from build123d import *

# Parameters (mm, degrees)
F2_R     = 2.54
F4_DEPTH = 3.81
F5_DEPTH = 5.08


with BuildPart() as f1:
    # F0 (on Front) → F1 (revolve)
    with BuildSketch(Plane.XZ):
        Polygon((0, 0), (0, 45.974), (-9.660285, 45.974), (-9.660285, 39.017074), (-6.224093, 36.049455), (-6.224093, 9.1948), (-8.699501, 9.1948), (-10.9982, 0), align=None)
    revolve(axis=Axis((0, 0, 22.987), (0, 0, 1)))

    # F2
    f2_edges = [f1.edges().sort_by_distance(p)[0] for p in [
        (8.699501, 0, 9.1948),
    ]]
    fillet(f2_edges, radius=F2_R)

    # F3 (on face) → F4 (cut)
    with BuildSketch(Plane.XY.offset(45.974)):
        with BuildLine():
            ThreePointArc((-5.499261, 3.175), (-4.490128, 4.490128), (-3.175, 5.499261))
            Line((-3.175, 5.499261), (-4.830143, 8.366052))
            ThreePointArc((-4.830143, 8.366052), (-6.830853, 6.830853), (-8.366052, 4.830143))
            Line((-8.366052, 4.830143), (-5.499261, 3.175))
        make_face()
        with BuildLine():
            ThreePointArc((0, 6.35), (1.643501, 6.133629), (3.175, 5.499261))
            Line((3.175, 5.499261), (4.830143, 8.366052))
            ThreePointArc((4.830143, 8.366052), (2.500266, 9.331119), (0, 9.660285))
            Line((0, 9.660285), (0, 6.35))
        make_face()
        with BuildLine():
            ThreePointArc((5.499261, 3.175), (6.133629, 1.643501), (6.35, 0))
            Line((6.35, 0), (9.660285, 0))
            ThreePointArc((9.660285, 0), (9.331119, 2.500266), (8.366052, 4.830143))
            Line((8.366052, 4.830143), (5.499261, 3.175))
        make_face()
        with BuildLine():
            Line((8.366052, -4.830143), (5.499261, -3.175))
            ThreePointArc((5.499261, -3.175), (4.490128, -4.490128), (3.175, -5.499261))
            Line((3.175, -5.499261), (4.830143, -8.366052))
            ThreePointArc((4.830143, -8.366052), (6.830853, -6.830853), (8.366052, -4.830143))
        make_face()
        with BuildLine():
            Line((0, -9.660285), (0, -6.35))
            ThreePointArc((0, -6.35), (-1.643501, -6.133629), (-3.175, -5.499261))
            Line((-3.175, -5.499261), (-4.830143, -8.366052))
            ThreePointArc((-4.830143, -8.366052), (-2.500266, -9.331119), (0, -9.660285))
        make_face()
        with BuildLine():
            Line((-8.366052, -4.830143), (-5.499261, -3.175))
            ThreePointArc((-5.499261, -3.175), (-6.133629, -1.643501), (-6.35, 0))
            Line((-6.35, 0), (-9.660285, 0))
            ThreePointArc((-9.660285, 0), (-9.331119, -2.500266), (-8.366052, -4.830143))
        make_face()
    extrude(amount=-F4_DEPTH, mode=Mode.SUBTRACT)

    # F3 (on face) → F5 (cut)
    with BuildSketch(Plane.XY.offset(45.974)):
        with BuildLine():
            ThreePointArc((5.499261, -3.175), (6.133629, -1.643501), (6.35, 0))
            ThreePointArc((6.35, 0), (6.133629, 1.643501), (5.499261, 3.175))
            ThreePointArc((5.499261, 3.175), (4.490128, 4.490128), (3.175, 5.499261))
            ThreePointArc((3.175, 5.499261), (1.643501, 6.133629), (0, 6.35))
            ThreePointArc((0, 6.35), (-1.643501, 6.133629), (-3.175, 5.499261))
            ThreePointArc((-3.175, 5.499261), (-4.490128, 4.490128), (-5.499261, 3.175))
            ThreePointArc((-5.499261, 3.175), (-6.133629, 1.643501), (-6.35, 0))
            ThreePointArc((-6.35, 0), (-6.133629, -1.643501), (-5.499261, -3.175))
            ThreePointArc((-5.499261, -3.175), (-4.490128, -4.490128), (-3.175, -5.499261))
            ThreePointArc((-3.175, -5.499261), (-1.643501, -6.133629), (0, -6.35))
            ThreePointArc((0, -6.35), (1.643501, -6.133629), (3.175, -5.499261))
            ThreePointArc((3.175, -5.499261), (4.490128, -4.490128), (5.499261, -3.175))
        make_face()
    extrude(amount=-F5_DEPTH, mode=Mode.SUBTRACT)


solid = f1.part
Read the model definition and answer for the solid it produces. Units are mm, in the model's axes. A direction names the side the tool comes from. Coordinates: 2 decimals unless noted, no trailing zeros. Loops run counter-clockwise (first coordinate to the right, second up) from the corner with the lowest first, then second, coordinate; pieces in that order, holes last. Notation, with made-up numbers: (88, -15) -> (102, -15) arc R15 ccw to (102, -10) -> close; hole circle Ø1 at (-12, 84.25). An arc over 180 degrees is marked (long way). Write item = value, one per line. Start each with the question number.
1) Find the intervals of material crossed by L1, parallel to Z at x = 4.75, y = -7.25; L2, parallel to Z at x = -1.25, y = 4.75; L3, parallel to Z at x = -4, y = 5, in increasing order. Write a range as from..to.
2) The mould has two halves that part along Z. Classify faces 1 (the face through (-3.99, -6.91, 44.1)), 2 (the face through (8, -2, 45.974)), 3 (the face through (1.385, 6.239, 36.194)): pulls with the +Z half, pulls with the -Z half, needs draft (parallel to the pull), parting line crosses it, or undercut.
3) The part is cut by section A-A, the plane z = 17.5. Determine the outline of the cut face in (x, y), plus the area to 3 significant figures.
4) Given P1, Ø1.5, axis at y = -5, z = 24.5, coming from the +X side; P2, Ø1.6, axis at x = -4.5, y = 6, coming from the +Z side; P3, Ø3.5, axis at y = 8.5, z = 43.5, coming from the +X side, each flat-ended and moving along its own axis, determine where each tip first touches the part or whether it passes through.
5) For faces 4 (the face through (1.349, 6.076, 22.434)), 5 (the face through (3.99, 6.91, 44.1)), 6 (the face through (-8.924, 3.7, 42.447)), 7 (the face through (-8, -2, 42.164)), 8 (the face through (0, -8, 44)), determine the directions among +Z, -Z, +X, -X, +Y, -Y from which every point of the face is accessible in a straight line to the end or side of a thin tool.
Result:
q1.L1 = 0..8.28, 38.16..42.16
q1.L2 = 0..40.89
q1.L3 = 0..9.19, 36.2..42.16
q2.face_1 = needs draft
q2.face_2 = pulls with the +Z half
q2.face_3 = undercut
q3.outline = circle Ø12.45 at (0, 0)
q3.area = 122 mm²
q4.P1 = 4.55
q4.P2 = 42.16
q4.P3 = 6.91
q5.face_4 = none
q5.face_5 = +Z, +Y
q5.face_6 = +Z
q5.face_7 = +Z, -X
q5.face_8 = +Z, -Y
